Model file for the job. Use its own axes, mm. A direction names the side the tool comes from. Round coordinates to 2 decimals unless told otherwise and drop trailing zeros. Loops run counter-clockwise (first coordinate to the right, second up) from the corner with the lowest first, then second, coordinate; pieces in that order, holes last. Notation, with made-up numbers: M 7,-29 L 61,-29 A10 ccw 61,-23 Z; hole C 86.5,4 d10. An arc over 180 degrees is marked long. Use a Markdown table: item, result. Add a question column.
Item 1: Saw through at D-D on x = 27.5. Write the cut outline in (y, z).
Item 2: Tool access for faces 1 (the cylindrical face through (-27.24, 11.71, 0.18)), 2 (the flat face through (2.54, -26, 0)), 3 (the flat face through (0, 6.477, -1)), 4 (the flat face through (-20.879, -12.096, -0.178)): list every direction of +Z, -Z, +X, -X, +Y, -Y with a clear straight run to the whole face (end or side of a thin tool).
Item 3: Saw through at C-C on z = 6.75. Give the number of separate pieces and of enclosed holes in the cut face, then the cut area to 3 significant figures.
Item 4: Saw through at B-B on x = 16.51. Write the cut outline in (y, z), then the cut area to 3 significant figures.
Item 5: Wall check: L1, parallel to Y at x = 0, z = 0.25; L2, parallel to X at y = 0, z = -3; L3, parallel to X at y = 16.51, z = -0.25. Give the ranges that are in metal, low to high. Write a range as from..to.
Item 6: Saw through at A-A on x = 0. Write the cut outline in (y, z).
Item 7: Pin check, flat tips, straight feed: P1, Ø1, axis at y = -25.5, z = 2, coming from the -X side; P2, Ø1, axis at y = -26, z = 6.5, coming from the +X side; P3, Ø3.5, axis at y = 26.5, z = -6, coming from the +X side; P4, Ø22, axis at x = -8.5, y = -10, coming from the +Z side. Stop position of each tip, or through.
```python
from build123d import *

# Parameters (mm, degrees)
SKETCH1_R                = 30.48
BOSS_EXTRUDE1_DEPTH      = 12.7
SKETCH2_R                = 31.75
BOSS_EXTRUDE2_DEPTH      = 1.27
SKETCH3_W                = 5.08
SKETCH3_H                = 7.62
CUT_EXTRUDE1_DEPTH       = 52.587643869
FILLET1_R                = 2.54
CIRPATTERN1_COUNT        = 6
FILLET1_OF_CIRPATTERN1_R = 2.54
CUT_EXTRUDE4_DEPTH       = 53.224648395
CUT_EXTRUDE4_DEPTH_BACK  = 53.224648395
SKETCH6_R                = 6.477
CUT_EXTRUDE5_DEPTH       = 53.224648395
CUT_EXTRUDE5_DEPTH_BACK  = 53.224648395
SKETCH7_R                = 1.778
SKETCH8_R                = 21.95890497
CUT_EXTRUDE6_DEPTH       = 1.016


with BuildPart() as part:
    # Sketch1 → Boss-Extrude1 (new, symmetric)
    with BuildSketch(Plane.XY):
        Circle(SKETCH1_R)
    extrude(amount=BOSS_EXTRUDE1_DEPTH, both=True)

    # Sketch2 → Boss-Extrude2 (add)
    with BuildSketch(Plane.XY.offset(-12.7)):
        Circle(SKETCH2_R)
    extrude(amount=-BOSS_EXTRUDE2_DEPTH)

    # Sketch3 → Cut-Extrude1 (cut, through all)
    with BuildSketch(Plane.XY.offset(-12.7)):
        with Locations((0, 27.94)):
            Rectangle(SKETCH3_W, SKETCH3_H)
    cut_extrude1 = extrude(amount=CUT_EXTRUDE1_DEPTH, mode=Mode.SUBTRACT)

    # Fillet1
    fillet1_edges = [part.edges().sort_by_distance(p)[0] for p in [
        (-2.54, 30.373982287, 0),
        (2.54, 30.373982287, 0),
    ]]
    fillet(fillet1_edges, radius=FILLET1_R)

    # CirPattern1: Cut-Extrude1 ×6 about axis
    cirpattern1_axis = Axis((0, 0, 0), (0, 0, 1))
    for i in range(1, CIRPATTERN1_COUNT):
        add(cut_extrude1.rotate(cirpattern1_axis, i * 360 / CIRPATTERN1_COUNT), mode=Mode.SUBTRACT)

    # Fillet1 of CirPattern1
    fillet1_of_cirpattern1_edges = [part.edges().sort_by_distance(p)[0] for p in [
        (-27.574640275, 12.987286618, 0),
        (-25.034640275, 17.386695669, 0),
        (-25.034640275, -17.386695669, 0),
        (-27.574640275, -12.987286618, 0),
        (2.54, -30.373982287, 0),
        (-2.54, -30.373982287, 0),
        (27.574640275, -12.987286618, 0),
        (25.034640275, -17.386695669, 0),
        (25.034640275, 17.386695669, 0),
        (27.574640275, 12.987286618, 0),
    ]]
    fillet(fillet1_of_cirpattern1_edges, radius=FILLET1_OF_CIRPATTERN1_R)

    # Sketch6 → Cut-Extrude4 (cut, two sides: drawn at the far end of the back side and taken through both)
    with BuildSketch(Plane(origin=(0, 0, -13.97), x_dir=(-1, 0, 0), z_dir=(0, 0, -1)).offset(-CUT_EXTRUDE4_DEPTH_BACK)):
        Circle(SKETCH6_R)
        with BuildLine():
            ThreePointArc((-5.609246563, -3.238499961), (-6.477, 1.38e-07), (-5.609246425, 3.2385002))
            Line((-5.609246425, 3.2385002), (-7.478995387, 0))
            Line((-7.478995387, 0), (-5.609246563, -3.238499961))
        make_face()
        with BuildLine():
            ThreePointArc((0, -6.477), (-3.23850002, -5.609246529), (-5.609246563, -3.238499961))
            Line((-5.609246563, -3.238499961), (-3.739497694, -6.477))
            Line((-3.739497694, -6.477), (0, -6.477))
        make_face()
        with BuildLine():
            ThreePointArc((5.609246485, -3.238500095), (3.238499952, -5.609246568), (0, -6.477))
            Line((0, -6.477), (3.739497694, -6.477))
            Line((3.739497694, -6.477), (5.609246485, -3.238500095))
        make_face()
        with BuildLine():
            Line((7.478995387, 0), (5.609246472, 3.238500118))
            ThreePointArc((5.609246472, 3.238500118), (6.256301559, 1.676371021), (6.477, 0))
            ThreePointArc((6.477, 0), (6.256301563, -1.676371008), (5.609246485, -3.238500095))
            Line((5.609246485, -3.238500095), (7.478995387, 0))
        make_face()
        with BuildLine():
            Line((3.739497694, 6.477), (2.1e-08, 6.477))
            ThreePointArc((2.1e-08, 6.477), (3.23849995, 5.609246569), (5.609246472, 3.238500118))
            Line((5.609246472, 3.238500118), (3.739497694, 6.477))
        make_face()
        with BuildLine():
            Line((2.1e-08, 6.477), (-3.739497694, 6.477))
            Line((-3.739497694, 6.477), (-5.609246425, 3.2385002))
            ThreePointArc((-5.609246425, 3.2385002), (-3.238499891, 5.609246603), (2.1e-08, 6.477))
        make_face()
    extrude(amount=CUT_EXTRUDE4_DEPTH + CUT_EXTRUDE4_DEPTH_BACK, mode=Mode.SUBTRACT)

    # Sketch7 → Cut-Extrude5 (cut, two sides: drawn at the far end of the back side and taken through both)
    with BuildSketch(Plane(origin=(0, 0, -13.97), x_dir=(-1, 0, 0), z_dir=(0, 0, -1)).offset(-CUT_EXTRUDE5_DEPTH_BACK)):
        with Locations((-16.51, 0)):
            Circle(SKETCH7_R)
        with Locations((0, 16.51)):
            Circle(SKETCH7_R)
        with Locations((16.51, 0)):
            Circle(SKETCH7_R)
        with Locations((0, -16.51)):
            Circle(SKETCH7_R)
    extrude(amount=CUT_EXTRUDE5_DEPTH + CUT_EXTRUDE5_DEPTH_BACK, mode=Mode.SUBTRACT)

    # Sketch8 → Cut-Extrude6 (cut)
    with BuildSketch(Plane(origin=(0, 0, 12.7), x_dir=(-1, 0, 0), z_dir=(0, 0, -1))):
        Circle(SKETCH8_R)
    extrude(amount=CUT_EXTRUDE6_DEPTH, mode=Mode.SUBTRACT)


solid = part.part
```
Entries:
| question | item | result |
|---|---|---|
| 1 | outline | M -15.87,-13.97 L 15.87,-13.97 L 15.87,-12.7 L 11.59,-12.7 L 11.59,12.7 L -11.59,12.7 L -11.59,-12.7 L -15.87,-12.7 Z |
| 2 | face 1 | +Z, +Y |
| 2 | face 2 | +Z, -Y |
| 2 | face 3 | +Z, -Z |
| 2 | face 4 | +Z |
| 3 | separate pieces | 1 |
| 3 | enclosed holes | 5 |
| 3 | area | 2,520 mm2 |
| 4 | outline | M -27.12,-13.97 L -1.78,-13.97 L -1.78,11.68 L -14.48,11.68 L -14.48,12.7 L -25.62,12.7 L -25.62,-12.7 L -27.12,-12.7 Z; M 1.78,-13.97 L 27.12,-13.97 L 27.12,-12.7 L 25.62,-12.7 L 25.62,12.7 L 14.48,12.7 L 14.48,11.68 L 1.78,11.68 Z |
| 4 | area | 1,250 mm2 |
| 5 | L1 | -24.13..-18.29, -14.73..-6.48, 6.48..14.73, 18.29..24.13 |
| 5 | L2 | -30.48..-18.29, -14.73..-7.48, 7.48..14.73, 18.29..30.48 |
| 5 | L3 | -23.2..-1.78, 1.78..23.2 |
| 6 | outline | M -31.75,-13.97 L -18.29,-13.97 L -18.29,11.68 L -21.96,11.68 L -21.96,12.7 L -24.13,12.7 L -24.13,-12.7 L -31.75,-12.7 Z; M -14.73,-13.97 L -6.48,-13.97 L -6.48,11.68 L -14.73,11.68 Z; M 6.48,-13.97 L 14.73,-13.97 L 14.73,11.68 L 6.48,11.68 Z; M 18.29,-13.97 L 31.75,-13.97 L 31.75,-12.7 L 24.13,-12.7 L 24.13,12.7 L 21.96,12.7 L 21.96,11.68 L 18.29,11.68 Z |
| 7 | P1 | x = -17.44 |
| 7 | P2 | x = 16.7 |
| 7 | P3 | x = 17.79 |
| 7 | P4 | z = 12.7 |
